Input: dimensioned drawing with shaded views. Units: mm. Origin: part minimum x, y, z. A direction names the side the tool comes from. Coordinates: 2 decimals unless noted, no trailing zeros. Write each loop counter-clockwise with the first axis right and the second up, starting at its lowest first coordinate (ties: lowest second). Pieces come first, ordered by that corner, then holes. Notation, with made-up numbers: (88, 13) -> (127, 13) arc R18 cw to (127, 34) -> close; hole circle Ø4 at (85, -5.5). An arc over 180 degrees is marked (long way). One line per item, written item: value. Start each with the question number.
1. Section query B-B, the plane x = 28. Output: boundary loops of the cut face in (y, z).
2. First-contact query: P1, Ø3.5, axis at x = 49.5, y = 49.5, coming from the -Z side; P2, Ø1.6, axis at x = 49, y = 7, coming from the -Z side; P3, Ø1, axis at x = 32, y = 20.5, coming from the -Z side; P4, Ø3, axis at x = 7, z = 10.5, coming from the +Y side. Flat tips, straight axial feed; report the tip coordinate or a pass-through.
3. Access query for the marked faces 1 and 2. Directions: +Z, -Z, +X, -X, +Y, -Y. A direction counts if a zero-diameter tool reaches every point of the face in a straight line with its end or side. Return the directions, or none.
4. Section query D-D, the plane y = 49.5. Output: boundary loops of the cut face in (x, z), and give its area (3 significant figures).
5. Section query A-A, the plane z = 18.25. Output: boundary loops of the cut face in (x, y).
6. Mould query, pull axis Y, two halves, no side actions, for the marked faces 3, 4 and 5. Classes: released by +Y, released by -Y, zero draft, split by the parting line, or undercut.
7. Line query: line 1 (Y direction, x = 6.5, z = 4); line 2 (Y direction, x = 6.5, z = 20.25). Output: solid intervals per line, ascending.
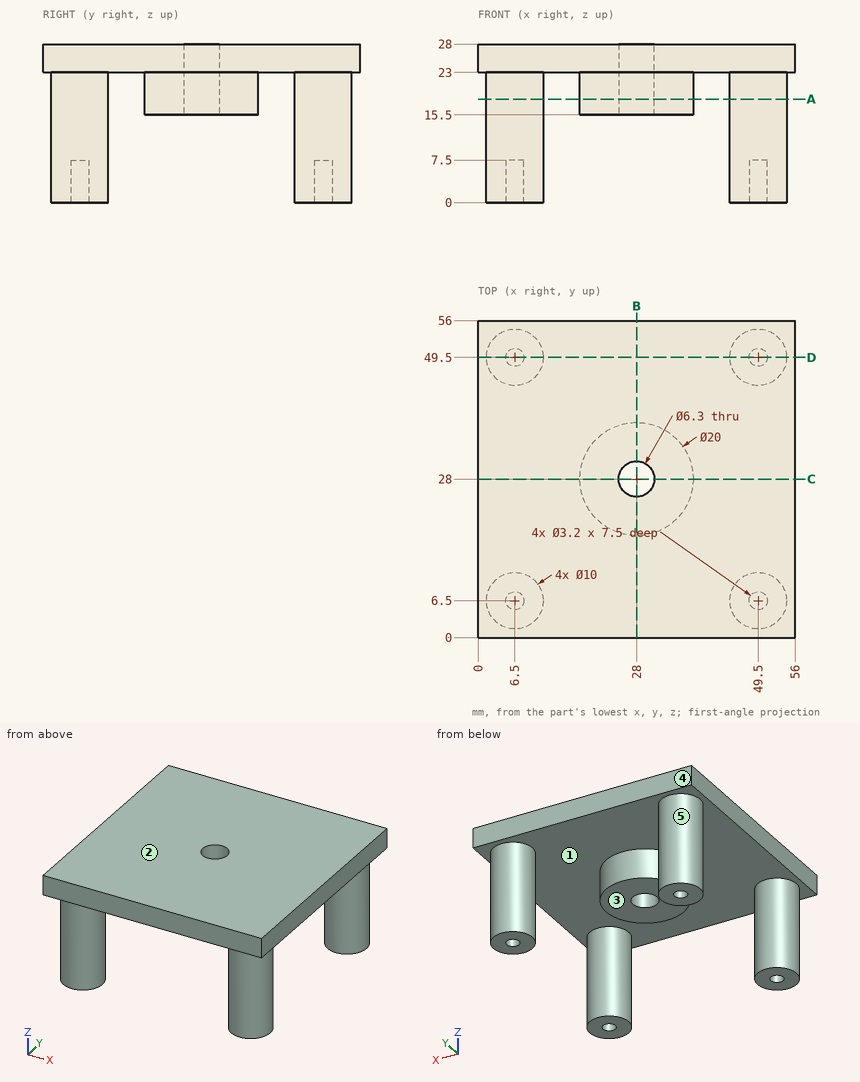
Computed values:
1. outline: (0, 23) -> (18, 23) -> (18, 15.5) -> (24.85, 15.5) -> (24.85, 28) -> (0, 28) -> close; (31.15, 15.5) -> (38, 15.5) -> (38, 23) -> (56, 23) -> (56, 28) -> (31.15, 28) -> close
2. P1: stops at z = 0
2. P2: stops at z = 7.5
2. P3: stops at z = 15.5
2. P4: stops at y = 54.5
3. face 1: -Z
3. face 2: +Z, +X, -X, +Y, -Y
4. outline: (0, 23) -> (1.5, 23) -> (1.5, 0) -> (4.9, 0) -> (4.9, 7.5) -> (8.1, 7.5) -> (8.1, 0) -> (11.5, 0) -> (11.5, 23) -> (44.5, 23) -> (44.5, 0) -> (47.9, 0) -> (47.9, 7.5) -> (51.1, 7.5) -> (51.1, 0) -> (54.5, 0) -> (54.5, 23) -> (56, 23) -> (56, 28) -> (0, 28) -> close
4. area: 692 mm²
5. outline: circle Ø10 at (6.5, 6.5); circle Ø10 at (6.5, 49.5); circle Ø20 at (28, 28); circle Ø10 at (49.5, 6.5); circle Ø10 at (49.5, 49.5); hole circle Ø6.3 at (28, 28)
6. face 3: zero draft
6. face 4: released by +Y
6. face 5: undercut
7. line 1: y = 1.5 to 4.9, 8.1 to 11.5, 44.5 to 47.9, 51.1 to 54.5
7. line 2: y = 1.5 to 11.5, 44.5 to 54.5
